```python
from build123d import *

# Parameters (mm, degrees)
SKETCH_R               = 2.425
PAD_DEPTH              = 12
POCKET_DEPTH           = 20
POCKET001_DEPTH        = 20
SKETCH003_R            = 1.5
POCKET002_DEPTH        = 20
SKETCH004_R            = 1.5
POCKET003_DEPTH        = 20
POCKET004_DEPTH        = 7
POCKET005_DEPTH        = 100
LINEARPATTERN_COUNT    = 2
LINEARPATTERN_PITCH    = 25
LINEARPATTERN001_COUNT = 2
LINEARPATTERN001_PITCH = 71
CHAMFER_SIZE           = 3
CHAMFER001_SIZE        = 10
CHAMFER002_SIZE        = 5


with BuildPart() as part:
    # Sketch → Pad (new body)
    with BuildSketch(Plane.XY):
        Polygon((-35.1, -47), (35.1, -47), (35.1, 48), (29.1, 48), (29.1, 89), (-35.1, 89), align=None)
        Circle(SKETCH_R, mode=Mode.SUBTRACT)
    extrude(amount=PAD_DEPTH)

    # Sketch001 (on Face9 of Pad) → Pocket (cut)
    with BuildSketch(Plane.XY.offset(12)):
        with BuildLine():
            ThreePointArc((11, 68), (0, 79), (-11, 68))
            Line((-11, 68), (-11, 58))
            ThreePointArc((-11, 58), (0, 47), (11, 58))
            Line((11, 58), (11, 68))
        make_face()
        with BuildLine():
            ThreePointArc((-14, 83.5), (-15.5, 85), (-17, 83.5))
            Line((-17, 83.5), (-17, 73.5))
            ThreePointArc((-17, 73.5), (-15.5, 72), (-14, 73.5))
            Line((-14, 73.5), (-14, 83.5))
        make_face()
        with BuildLine():
            ThreePointArc((-14, 52.5), (-15.5, 54), (-17, 52.5))
            Line((-17, 52.5), (-17, 42.5))
            ThreePointArc((-17, 42.5), (-15.5, 41), (-14, 42.5))
            Line((-14, 42.5), (-14, 52.5))
        make_face()
        with BuildLine():
            ThreePointArc((17, 83.5), (15.5, 85), (14, 83.5))
            Line((14, 83.5), (14, 73.5))
            ThreePointArc((14, 73.5), (15.5, 72), (17, 73.5))
            Line((17, 73.5), (17, 83.5))
        make_face()
    extrude(amount=-POCKET_DEPTH, mode=Mode.SUBTRACT)

    # Sketch002 (on Face5 of Pocket) → Pocket001 (cut)
    with BuildSketch(Plane.XY.offset(12)):
        with BuildLine():
            ThreePointArc((27.1, 75), (25.1, 77), (23.1, 75))
            Line((23.1, 75), (23.1, 51))
            ThreePointArc((23.1, 51), (25.1, 49), (27.1, 51))
            Line((27.1, 51), (27.1, 75))
        make_face()
    extrude(amount=-POCKET001_DEPTH, mode=Mode.SUBTRACT)

    # Sketch003 (on Face5 of Pocket001) → Pocket002 (cut)
    with BuildSketch(Plane.XY.offset(12)):
        with Locations((-31.78, 62.85)):
            Circle(SKETCH003_R)
        with Locations((-31.78, 43.85)):
            Circle(SKETCH003_R)
    extrude(amount=-POCKET002_DEPTH, mode=Mode.SUBTRACT)

    # Sketch004 (on Face5 of Pocket002) → Pocket003 (cut)
    with BuildSketch(Plane.XY.offset(12)):
        with Locations((14.999119, 47.004734)):
            Circle(SKETCH004_R)
    extrude(amount=-POCKET003_DEPTH, mode=Mode.SUBTRACT)

    # Sketch005 (on Face5 of Pocket003) → Pocket004 (cut)
    with BuildSketch(Plane.XY.offset(12)):
        Polygon((14.999119, 43.887043), (17.699119, 45.445888), (17.699119, 48.56358), (14.999119, 50.122425), (12.299119, 48.56358), (12.299119, 45.445888), align=None)
    extrude(amount=-POCKET004_DEPTH, mode=Mode.SUBTRACT)

    # Sketch006 (on Face3 of Pocket004) → Pocket005 (cut)
    with BuildSketch(Plane.YZ.offset(35.1)):
        with BuildLine():
            ThreePointArc((-38.180538, 6.552041), (-38.95, 5), (-38.180538, 3.447959))
            Line((-38.180538, 3.447959), (-37, 2.55))
            Line((-37, 2.55), (-35.819462, 3.447959))
            ThreePointArc((-35.819462, 3.447959), (-35.05, 5), (-35.819462, 6.552041))
            Line((-37, 7.45), (-35.819462, 6.552041))
            Line((-37, 7.45), (-38.180538, 6.552041))
        make_face()
    pocket005 = extrude(amount=-POCKET005_DEPTH, mode=Mode.SUBTRACT)

    # LinearPattern: Pocket005 ×2
    with Locations(*[(0, i * LINEARPATTERN_PITCH, 0) for i in range(1, LINEARPATTERN_COUNT)]):
        add(pocket005, mode=Mode.SUBTRACT)

    # LinearPattern001: Pocket005 ×2
    with Locations(*[(0, i * LINEARPATTERN001_PITCH, 0) for i in range(1, LINEARPATTERN001_COUNT)]):
        add(pocket005, mode=Mode.SUBTRACT)

    # Chamfer
    chamfer_edges = [part.edges().sort_by_distance(p)[0] for p in [
        (29.1, 48, 6),
    ]]
    chamfer(chamfer_edges, length=CHAMFER_SIZE)

    # Chamfer001
    chamfer001_edges = [part.edges().sort_by_distance(p)[0] for p in [
        (29.1, 89, 6),
    ]]
    chamfer(chamfer001_edges, length=CHAMFER001_SIZE)

    # Chamfer002
    chamfer002_edges = [part.edges().sort_by_distance(p)[0] for p in [
        (-35.1, 89, 6),
    ]]
    chamfer(chamfer002_edges, length=CHAMFER002_SIZE)


solid = part.part
```
Can you work these out from the model? Positions are in its coordinate system, mm. A direction names the side the tool comes from. Give positions to 0.01 mm unless a question says otherwise; leave off trailing zeros. Order: outer loops, then holes, each group sorted by start corner. A loop starts at its lowest first (then second) coordinate and runs counter-clockwise, first axis right, second up. Notation, with made-up numbers: M 81.5,-15 L 122.5,-15 A3 ccw 122.5,-10 Z; hole C 49,88.25 d11. An arc over 180 degrees is marked long. One line per item, written item: value.
1) I want a section at A-A, the plane x = -15.5. Count the separate pieces of the cut face and the enclosed holes in it, plus the area to 3 significant figures.
Answer sheet:
separate pieces: 3
enclosed holes: 3
area: 1,280 mm^2
2) Please list where these lines run through material, in increasing order: line 1 along X through (y, z) = (51.5, 4.25); line 2 along Y through (x, z) = (15, 9.75); line 3 along Y through (x, z) = (-21.5, 4.5).
Answer sheet:
line 1: x = -35.1 to -17, -14 to -8.87, 8.87 to 23.1, 27.1 to 29.1
line 2: y = -47 to 43.89, 50.12 to 72.09, 84.91 to 89
line 3: y = -47 to -38.88, -35.12 to -13.88, -10.12 to 32.12, 35.88 to 89
3) I want a section at B-B, the plane y = 0. List the corners of the cut face in (x, z) for me (3 decimals), plus the area to 3 significant figures.
Answer sheet:
outline: M -35.1,0 L -2.425,0 L -2.425,12 L -35.1,12 Z; M 2.425,0 L 35.1,0 L 35.1,12 L 2.425,12 Z
area: 784 mm^2
4) For P1, Ø2.5, axis at x = 15.5, y = 48, coming from the +Z side; P2, Ø3, axis at y = 76, z = 4.5, coming from the +X side, each with a flat end and sliding along its axis, tell me the tip position at first contact or that it passes through.
Answer sheet:
P1: stops at z = 5
P2: stops at x = 29.1
5) We'd pull the mould along X, two halves only. Please class faces 1 (the face through (25.1, 77, 6.1)), 2 (the face through (-35.1, 19, 6)), 3 (the face through (34, 48, 6)): released by +X, released by -X, zero draft, split by the parting line, or undercut.
Answer sheet:
face 1: undercut
face 2: released by -X
face 3: zero draft
6) On a 3-axis mill with a long thin cutter (end or side, diameter ignored), from which of +Z, -Z, +X, -X, +Y, -Y can I reach the whole of each face in a straight line? I mean faces 4 (the face through (30.6, 49.5, 5.9)), 5 (the face through (0.49, 32.05, 5.03)), 6 (the face through (-11, 63, 6)), 7 (the face through (17.699, 47, 9)). Say none if no direction works.
Answer sheet:
face 4: +Z, -Z, +X, +Y
face 5: +X, -X
face 6: +Z, -Z
face 7: +Z
7) I want a section at C-C, the plane x = 25.1. List the corners of the cut face in (y, z) for me, plus the area to 3 significant figures.
Answer sheet:
outline: M -47,0 L 49,0 L 49,12 L -47,12 Z; M 77,0 L 83,0 L 83,12 L 77,12 Z; hole M -38.18,3.45 L -37,2.55 L -35.82,3.45 A1.95 ccw -35.82,6.55 L -37,7.45 L -38.18,6.55 A1.95 ccw Z; hole M -13.18,3.45 L -12,2.55 L -10.82,3.45 A1.95 ccw -10.82,6.55 L -12,7.45 L -13.18,6.55 A1.95 ccw Z; hole M 32.82,3.45 L 34,2.55 L 35.18,3.45 A1.95 ccw 35.18,6.55 L 34,7.45 L 32.82,6.55 A1.95 ccw Z
area: 1,190 mm^2
8) I want a section at D-D, the plane x = -26. List the corners of the cut face in (y, z) for me.
Answer sheet:
outline: M -47,0 L 89,0 L 89,12 L -47,12 Z; hole M -38.18,3.45 L -37,2.55 L -35.82,3.45 A1.95 ccw -35.82,6.55 L -37,7.45 L -38.18,6.55 A1.95 ccw Z; hole M -13.18,3.45 L -12,2.55 L -10.82,3.45 A1.95 ccw -10.82,6.55 L -12,7.45 L -13.18,6.55 A1.95 ccw Z; hole M 32.82,3.45 L 34,2.55 L 35.18,3.45 A1.95 ccw 35.18,6.55 L 34,7.45 L 32.82,6.55 A1.95 ccw Z
